Can you work these out from the model? Positions are in its coordinate system, mm. A direction names the side the tool comes from. Round coordinates to 2 decimals unless told otherwise and drop trailing zeros. Loops run counter-clockwise (first coordinate to the right, second up) from the corner with the lowest first, then second, coordinate; pieces in that order, holes last. Notation, with made-up numbers: (63, 11.5) -> (111, 11.5) arc R21 ccw to (111, 39.5) -> close; hole circle Ø2 at (-40, -9). An arc over 180 degrees is marked (long way). Answer as a JSON object with one key per item and string values.
```python
from build123d import *

# Parameters (mm, degrees)
CROQUIS1_R                   = 2.9
CROQUIS1_R_2                 = 2
SALIENTE_EXTRUIR1_DEPTH      = 3.9
SALIENTE_EXTRUIR2_DEPTH      = 3.9
SALIENTE_EXTRUIR2_DEPTH_BACK = 3.9
REDONDEO1_R                  = 5


with BuildPart() as part:
    # Croquis1 → Saliente-Extruir1 (new body)
    with BuildSketch(Plane(origin=(0, 0, 0), x_dir=(1, 0, 0), z_dir=(0, 1, 0))):
        with Locations(Location((0, 0, 0), (0, 0, 270))):
            Circle(CROQUIS1_R)
        with Locations(Location((0, 0, 0), (0, 0, 270))):
            Circle(CROQUIS1_R_2, mode=Mode.SUBTRACT)
    extrude(amount=SALIENTE_EXTRUIR1_DEPTH)

    # Croquis2 → Saliente-Extruir2 (add, two sides: drawn at the far end of the back side and taken through both)
    with BuildSketch(Plane.XZ.offset(-SALIENTE_EXTRUIR2_DEPTH_BACK)):
        with BuildLine():
            Line((-45, -2.9), (0, -2.9))
            ThreePointArc((0, -2.9), (-1.702938637, -2.347338919), (-2.75680975, -0.9))
            Line((-2.75680975, -0.9), (-45, -0.9))
            Line((-45, -0.9), (-45, -2.9))
        make_face()
    extrude(amount=SALIENTE_EXTRUIR2_DEPTH + SALIENTE_EXTRUIR2_DEPTH_BACK)

    # Redondeo1
    # the kernel refuses this fillet: 5 mm, written as the material it takes off along each edge
    with BuildSketch(Plane(origin=(-45, 13.9, -0.9), x_dir=(0, 0, -1), z_dir=(0, -1, 0))) as redondeo1_piece_1:
        with BuildLine():
            CenterArc((5, 4), REDONDEO1_R, 180, 53.130102354)
            Line((0, 4), (-0.1, 4))
            Line((-0.1, 4), (-0.1, 0))
            Line((-0.1, 0), (0, -0.1))
            ThreePointArc((0, -0.1), (1, -0.1), (1.94, -0.08))
            Line((1.94, -0.08), (2, 0))
        make_face()
    extrude(amount=27.8, mode=Mode.SUBTRACT)


solid = part.part
```
Q1. I'm going to push flat-ended pins straight in: pin 1 (3 mm diameter, centred on x = -1, z = 0, fed in from -Y); pin 2 (4 mm diameter, centred on x = -32, y = 2, fed in from +Z); pin 3 (1.5 mm diameter, centred on y = 2.5, z = 1.5, fed in from +X). Where does each tip first touch, or does it pass through?
Determined:
{"pin 1": "y = 0", "pin 2": "z = -0.9", "pin 3": "x = 2.8"}
Q2. If I drill on L1, parallel to X at y = 2, z = 0; L2, parallel to X at y = 2.5, z = 1.8; L3, parallel to Z at x = -28, y = 2.5, over which ranges is the centre line in solid material (lowest first)? Write a range as [from, to].
Determined:
{"L1": "[-2.9, -2], [2, 2.9]", "L2": "[-2.27, -0.87], [0.87, 2.27]", "L3": "[-2.9, -0.9]"}
Q3. On a 3-axis mill with a long thin cutter (end or side, diameter ignored), from which of +Z, -Z, +X, -X, +Y, -Y can I reach the whole of each face in a straight line? I mean faces 1 (the cylindrical face through (-1.682, -1.923, -2.362)), 2 (the flat face through (-19, 3.9, -2)). Say none if no direction works.
Determined:
{"face 1": "+Z, +X, -Y", "face 2": "+Z, -Z, +X, -X, +Y"}
Q4. I want a section at D-D, the plane x = -23. Write out the boundary of the cut face in (y, z), then the cut area to 3 significant figures.
Determined:
{"outline": "(-3.9, -2.9) -> (3.9, -2.9) -> (3.9, -0.9) -> (-3.9, -0.9) -> close", "area": "15.6 mm²"}
Q5. We'd pull the mould along Z, two halves only. Please class faces 3 (the flat face through (-2, 0, -1)), 4 (the cylindrical face through (-2, 2, 0)), 5 (the flat face through (-23, 0, -2.9)): pulls with the +Z half, pulls with the -Z half, needs draft (parallel to the pull), parting line crosses it, or undercut.
Determined:
{"face 3": "needs draft", "face 4": "undercut", "face 5": "pulls with the -Z half"}
Q6. I want a section at B-B, the plane y = 1.75. Write out the boundary of the cut face in (x, z).
Determined:
{"outline": "(-45, -2.9) -> (0, -2.9) arc R2.9 ccw (long way) to (-2.76, -0.9) -> (-41, -0.9) arc R5 ccw to start; hole circle Ø4 at (0, 0)"}
Q7. I want a section at A-A, the plane z = 0. Write out the boundary of the cut face in (x, y).
Determined:
{"outline": "(-2.9, 0) -> (-2, 0) -> (-2, 3.9) -> (-2.9, 3.9) -> close; (2, 0) -> (2.9, 0) -> (2.9, 3.9) -> (2, 3.9) -> close"}
Q8. I want a section at C-C, the plane y = -2.75. Write out the boundary of the cut face in (x, z).
Determined:
{"outline": "(-45, -2.9) -> (0, -2.9) arc R2.9 cw to (-2.76, -0.9) -> (-41, -0.9) arc R5 ccw to start"}
